Can you work these out from the model? Positions are in its coordinate system, mm. Face numbers are marked on the shaded views. A direction names the side the tool comes from. Give positions to 0.01 mm unless a question says otherwise; leave off trailing zeros. Loops run counter-clockwise (first coordinate to the right, second up) from the corner with the lowest first, then second, coordinate; pieces in that order, holes last. Notation, with made-up numbers: M 42,-20.75 L 50,-20.75 A21 cw 50,-14.75 Z; hole C 59,83 d6. An arc over 180 degrees is marked long. Answer as a JSON object with one key per item and string values.
```python
from build123d import *

# Parameters (mm, degrees)
SKETCH_1_R          = 1
EXTRUDE_1_DEPTH     = 6
SKETCH_2_R          = 2.25
EXTRUDE_2_DEPTH     = 1
SKETCH_3_W          = 2.5
SKETCH_3_H          = 0.75
CUT_EXTRUDE_1_DEPTH = 0.5
SKETCH_4_W          = 0.75
SKETCH_4_H          = 2.5
CUT_EXTRUDE_2_DEPTH = 0.5


with BuildPart() as part:
    # 草图1 → 拉伸1 (new body)
    with BuildSketch(Plane(origin=(0, 0, 0), x_dir=(1, 0, 0), z_dir=(0, 1, 0))):
        with Locations(Location((0, 0, 0), (0, 0, 270))):
            Circle(SKETCH_1_R)
    extrude(amount=EXTRUDE_1_DEPTH)

    # 草图2 → 拉伸2 (add)
    with BuildSketch(Plane(origin=(0, 6, 0), x_dir=(-1, 0, 0), z_dir=(0, 1, 0))):
        with Locations(Location((0, 0, 0), (0, 0, 90))):
            Circle(SKETCH_2_R)
    extrude(amount=EXTRUDE_2_DEPTH)

    # 草图3 → 切除-拉伸1 (cut)
    with BuildSketch(Plane(origin=(0, 7, 0), x_dir=(-1, 0, 0), z_dir=(0, 1, 0))):
        Rectangle(SKETCH_3_W, SKETCH_3_H)
    extrude(amount=-CUT_EXTRUDE_1_DEPTH, mode=Mode.SUBTRACT)

    # 草图4 → 切除-拉伸2 (cut)
    with BuildSketch(Plane(origin=(0, 7, 0), x_dir=(-1, 0, 0), z_dir=(0, 1, 0))):
        Rectangle(SKETCH_4_W, SKETCH_4_H)
    extrude(amount=-CUT_EXTRUDE_2_DEPTH, mode=Mode.SUBTRACT)


solid = part.part
```
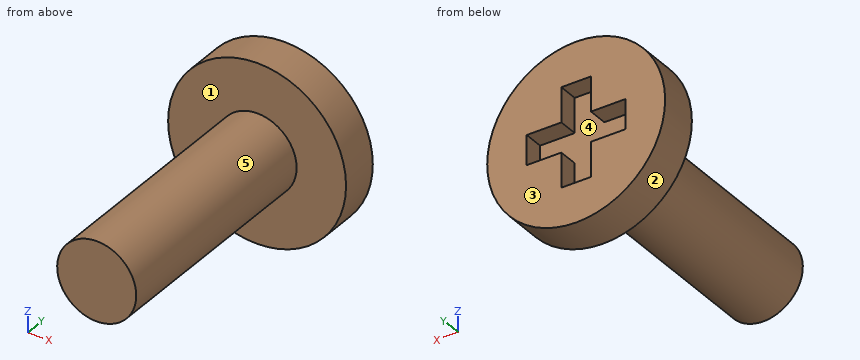
1) If we mould it in two halves opening along Z, with no side actions, what happens to the marked faces 3, 4 and 5? For each: +Z half, -Z half, draft (parallel to the pull), parting line (faces both ways), or undercut.
Answer list:
{"face 3": "draft", "face 4": "undercut", "face 5": "parting line"}
2) Suppose I cut it at D-D, the plane y = 6.25. Write out the boundary of the cut face in (x, z).
Answer list:
{"outline": "C 0,0 d4.5"}
3) Please list where these lines run through material, in increasing order: line 1 along X through (y, z) = (3.75, 0); line 2 along Y through (x, z) = (-1.05, -0.95); line 3 along X through (y, z) = (6.25, 0.1). Write a range as from..to.
Answer list:
{"line 1": "-1..1", "line 2": "6..7", "line 3": "-2.25..2.25"}
4) For the marked faces 1 and 2, which set-ups out of +Z, -Z, +X, -X, +Y, -Y let a thin tool reach every point of the face, with its end or its side?
Answer list:
{"face 1": "-Y", "face 2": "+Y, -Y"}
5) Will these pins go through, and if not, where does the flat tip stop? pin 1 Ø0.6 at (y, z) = (6.5, 1) entering from +X; pin 2 Ø1.5 at (x, y) = (0, 3) entering from -Z; pin 3 Ø0.6 at (x, y) = (-1, 6.5) entering from +Z.
Answer list:
{"pin 1": "x = 2.14", "pin 2": "z = -1", "pin 3": "z = 2.14"}
6) Suppose I cut it at A-A, the plane x = 0. Write out the boundary of the cut face in (y, z).
Answer list:
{"outline": "M 0,-1 L 6,-1 L 6,-2.25 L 7,-2.25 L 7,-1.25 L 6.5,-1.25 L 6.5,1.25 L 7,1.25 L 7,2.25 L 6,2.25 L 6,1 L 0,1 Z"}
7) Suppose I cut it at B-B, the plane z = 0. Write out the boundary of the cut face in (x, y).
Answer list:
{"outline": "M -2.25,6 L -1,6 L -1,0 L 1,0 L 1,6 L 2.25,6 L 2.25,7 L 1.25,7 L 1.25,6.5 L -1.25,6.5 L -1.25,7 L -2.25,7 Z"}
8) Suppose I cut it at C-C, the plane y = 2. Write out the boundary of the cut face in (x, z), and give its area (3 significant figures).
Answer list:
{"outline": "C 0,0 d2", "area": "3.14 mm^2"}
